```python
from build123d import *

# Parameters (mm, degrees)
SKETCH1_R           = 0.85
BOSS_EXTRUDE1_DEPTH = 3


with BuildPart() as part:
    # Sketch1 → Boss-Extrude1 (new body)
    with BuildSketch(Plane.XY):
        with BuildLine():
            Line((-1.045955351, 4.889373927), (-0.5, 6.389373927))
            Line((-0.5, 6.389373927), (0.5, 6.389373927))
            Line((0.5, 6.389373927), (1.045955351, 4.889373927))
            ThreePointArc((1.045955351, 4.889373927), (1.545084972, 4.755282581), (2.027706233, 4.570383729))
            Line((2.027706233, 4.570383729), (3.351071269, 5.463004717))
            Line((3.351071269, 5.463004717), (4.160088263, 4.875219465))
            Line((4.160088263, 4.875219465), (3.720097542, 3.340789469))
            ThreePointArc((3.720097542, 3.340789469), (4.045084972, 2.938926261), (4.326852955, 2.505662288))
            Line((4.326852955, 2.505662288), (5.922147212, 2.449953385))
            Line((5.922147212, 2.449953385), (6.231164206, 1.498896869))
            Line((6.231164206, 1.498896869), (4.973288913, 0.516136983))
            ThreePointArc((4.973288913, 0.516136983), (5, 0), (4.973288913, -0.516136983))
            Line((4.973288913, -0.516136983), (6.231164206, -1.498896869))
            Line((6.231164206, -1.498896869), (5.922147212, -2.449953385))
            Line((5.922147212, -2.449953385), (4.326852955, -2.505662288))
            ThreePointArc((4.326852955, -2.505662288), (4.045084972, -2.938926261), (3.720097542, -3.340789469))
            Line((3.720097542, -3.340789469), (4.160088263, -4.875219465))
            Line((4.160088263, -4.875219465), (3.351071269, -5.463004717))
            Line((3.351071269, -5.463004717), (2.027706233, -4.570383729))
            ThreePointArc((2.027706233, -4.570383729), (1.545084972, -4.755282581), (1.045955351, -4.889373927))
            Line((1.045955351, -4.889373927), (0.5, -6.389373927))
            Line((0.5, -6.389373927), (-0.5, -6.389373927))
            Line((-0.5, -6.389373927), (-1.045955351, -4.889373927))
            ThreePointArc((-1.045955351, -4.889373927), (-1.545084972, -4.755282581), (-2.027706233, -4.570383729))
            Line((-2.027706233, -4.570383729), (-3.351071269, -5.463004717))
            Line((-3.351071269, -5.463004717), (-4.160088263, -4.875219465))
            Line((-4.160088263, -4.875219465), (-3.720097542, -3.340789469))
            ThreePointArc((-3.720097542, -3.340789469), (-4.045084972, -2.938926261), (-4.326852955, -2.505662288))
            Line((-4.326852955, -2.505662288), (-5.922147212, -2.449953385))
            Line((-5.922147212, -2.449953385), (-6.231164206, -1.498896869))
            Line((-6.231164206, -1.498896869), (-4.973288913, -0.516136983))
            ThreePointArc((-4.973288913, -0.516136983), (-5, 0), (-4.973288913, 0.516136983))
            Line((-4.973288913, 0.516136983), (-6.231164206, 1.498896869))
            Line((-6.231164206, 1.498896869), (-5.922147212, 2.449953385))
            Line((-5.922147212, 2.449953385), (-4.326852955, 2.505662288))
            ThreePointArc((-4.326852955, 2.505662288), (-4.045084972, 2.938926261), (-3.720097542, 3.340789469))
            Line((-3.720097542, 3.340789469), (-4.160088263, 4.875219465))
            Line((-4.160088263, 4.875219465), (-3.351071269, 5.463004717))
            Line((-3.351071269, 5.463004717), (-2.027706233, 4.570383729))
            ThreePointArc((-2.027706233, 4.570383729), (-1.545084972, 4.755282581), (-1.045955351, 4.889373927))
        make_face()
        Circle(SKETCH1_R, mode=Mode.SUBTRACT)
    extrude(amount=BOSS_EXTRUDE1_DEPTH)


solid = part.part
```
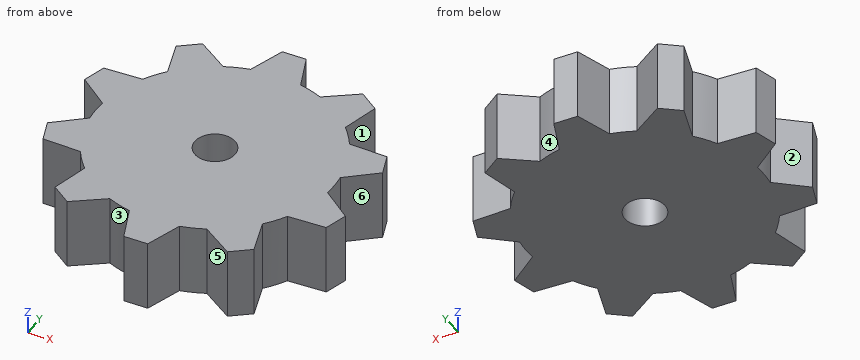
Model file for the job. Use its own axes, mm. Face numbers are marked on the shaded views. A direction names the side the tool comes from. Give positions to 0.01 mm unless a question says otherwise; leave off trailing zeros. Order: outer loops, then holes, each group sorted by start corner. A loop starts at its lowest first (then second) coordinate and runs counter-clockwise, first axis right, second up.
1) Mould opens along X. For the marked faces 1, 2 and 3 say: +X half, -X half, draft (parallel to the pull), parting line (faces both ways), or undercut.
2) Wall check: probe 1 along Y at (x, z) = (0, 2.2); probe 2 along X at (y, z) = (5, 2.05); probe 3 along X at (y, z) = (-0.75, 1.35). Give the ranges that are in metal, low to high.
3) Saw through at C-C, the plane x = -3.5. Write the cut outline in (y, z), then the cut area to 3 significant figures.
4) Pin check, flat tips, straight feed: pin 1 (2 mm diameter, centred on x = 0, y = 0, fed in from +Z); pin 2 (1.5 mm diameter, centred on x = -2.5, z = 1, fed in from -Y). Stop position of each tip, or through.
5) 3-axis set-ups, long thin cutter, end or side, ignore diameter. For the marked faces 4, 5 and 6: which of +Z, -Z, +X, -X, +Y, -Y reach the whole face in a straight line?
6) Saw through at B-B, the plane y = 0. Write the cut outline in (x, z).
7) Saw through at A-A, the plane x = 0. Write the cut outline in (y, z).
8) Saw through at D-D, the plane x = -1.25. Write the cut outline in (y, z).
Computed:
1. face 1: +X half
1. face 2: -X half
1. face 3: undercut
2. probe 1: y = -6.39 to -0.85, 0.85 to 6.39
2. probe 2: x = -3.99 to -2.66, -1.01 to 1.01, 2.66 to 3.99
2. probe 3: x = -5.27 to -0.4, 0.4 to 5.27
3. outline: (-5.35, 0) - (5.35, 0) - (5.35, 3) - (-5.35, 3) - close
3. area: 32.1 mm2
4. pin 1: stops at z = 3
4. pin 2: stops at y = -5.39
5. face 4: +Z, -Z, +Y
5. face 5: +Z, -Z, -Y
5. face 6: +Z, -Z, +X
6. outline: (-5, 0) - (-0.85, 0) - (-0.85, 3) - (-5, 3) - close; (0.85, 0) - (5, 0) - (5, 3) - (0.85, 3) - close
7. outline: (-6.39, 0) - (-0.85, 0) - (-0.85, 3) - (-6.39, 3) - close; (0.85, 0) - (6.39, 0) - (6.39, 3) - (0.85, 3) - close
8. outline: (-4.84, 0) - (4.84, 0) - (4.84, 3) - (-4.84, 3) - close
